from build123d import *

# Parameters (mm, degrees)
SKETCH_2_W               = 14
SKETCH_2_H               = 8
EXTRUDE_2_DEPTH          = 9
CUT_EXTRUDE_1_DEPTH      = 13.083045974
CUT_EXTRUDE_1_DEPTH_BACK = 13.083045974
SKETCH_3_R               = 1.35
SKETCH_3_2_R             = 1.35
EXTRUDE_3_DEPTH          = 3
SKETCH_6_R               = 1.5
CUT_EXTRUDE_3_DEPTH      = 10
SKETCH_7_R               = 4.5
CUT_EXTRUDE_4_DEPTH      = 4


with BuildPart() as part:
    # Sketch 2 → Extrude 2 (new, symmetric)
    with BuildSketch(Plane.XY):
        Rectangle(SKETCH_2_W, SKETCH_2_H)
    extrude(amount=EXTRUDE_2_DEPTH, both=True)

    # Sketch 3 → Cut-Extrude 1 (cut, two sides: drawn at the far end of the back side and taken through both)
    with BuildSketch(Plane(origin=(0, 0, 0), x_dir=(0, 0, -1), z_dir=(1, 0, 0)).offset(-CUT_EXTRUDE_1_DEPTH_BACK)):
        with Locations((6, 0)):
            Circle(SKETCH_3_R)
        with Locations((-6, 0)):
            Circle(SKETCH_3_R)
    extrude(amount=CUT_EXTRUDE_1_DEPTH + CUT_EXTRUDE_1_DEPTH_BACK, mode=Mode.SUBTRACT)

    # Sketch 3_2 → Extrude 3 (add, symmetric)
    with BuildSketch(Plane(origin=(0, 0, 0), x_dir=(0, 0, -1), z_dir=(1, 0, 0))):
        with Locations((6, 0)):
            Circle(SKETCH_3_2_R)
        with Locations((-6, 0)):
            Circle(SKETCH_3_2_R)
    extrude(amount=EXTRUDE_3_DEPTH, both=True)

    # Sketch 6 → Cut-Extrude 3 (cut)
    with BuildSketch(Plane.XZ.offset(4)):
        with Locations(Location((0, 0, 0), (0, 0, 270))):
            Circle(SKETCH_6_R)
    extrude(amount=-CUT_EXTRUDE_3_DEPTH, mode=Mode.SUBTRACT)

    # Sketch 7 → Cut-Extrude 4 (cut)
    with BuildSketch(Plane.XZ.offset(-4)):
        with Locations(Location((0, 0, 0), (0, 0, 270))):
            Circle(SKETCH_7_R)
    extrude(amount=CUT_EXTRUDE_4_DEPTH, mode=Mode.SUBTRACT)


solid = part.part
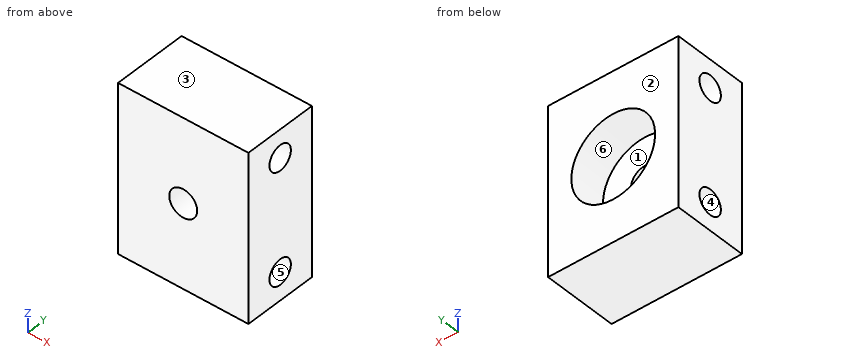
Read the model definition and answer for the solid it produces. Units are mm, in the model's axes. Face numbers are marked on the shaded views. A direction names the side the tool comes from. Give positions to 0.01 mm unless a question says otherwise; leave off trailing zeros. Write each loop counter-clockwise with the first axis right and the second up, starting at its lowest first coordinate (ties: lowest second). Pieces come first, ordered by that corner, then holes. Notation, with made-up numbers: (64.25, 7) - (85.25, 7) arc R13 cw to (85.25, 12) - close; hole circle Ø7 at (11, 50.5). An arc over 180 degrees is marked (long way). Use CSV: the item, a comma, the result in double quotes. Start each with the question number.
Item 1: For the marked faces 4, 5 and 6, determine the directions among +Z, -Z, +X, -X, +Y, -Y from which every point of the face is accessible in a straight line to the end or side of a thin tool.
Item 2: The part is cut by section C-C, the plane y = 2.5. Give the vertices of the cut face in (x, z).
Item 3: Flat-ended cylindrical pins translate along their axes: P1, Ø7, axis at x = 0, z = 0, coming from the -Y side; P2, Ø1.3, axis at y = 0, z = -6.5, coming from the +X side; P3, Ø2, axis at y = 0, z = -6, coming from the -X side. Find the tip coordinate at first contact, or state that the pin passes through.
Item 4: The part is cut by section B-B, the plane x = 0. Give the vertices of the cut face in (y, z), and give its area (3 significant figures).
Item 5: Consider line 1 (Z direction, x = 6.15, y = 0); line 2 (X direction, y = -0.5, z = 0); line 3 (Y direction, x = -5.3, z = 6). Determine where each line is inside the solid, lowest interval first.
Item 6: The part is cut by section D-D, the plane z = -6. Give the vertices of the cut face in (x, y).
Item 7: The part is cut by section A-A, the plane z = 0. Give the vertices of the cut face in (x, y).
Item 8: The mould has two halves that part along Z. Classify the marked faces 1, 2 and 3: pulls with the +Z half, pulls with the -Z half, needs draft (parallel to the pull), parting line crosses it, or undercut.
Taken from the geometry:
1,face 4,"-X"
1,face 5,"+X"
1,face 6,"+Y"
2,outline,"(-7, -9) - (7, -9) - (7, 9) - (-7, 9) - close; hole circle Ø9 at (0, 0)"
3,P1,"y = -4"
3,P2,"x = 3"
3,P3,"x = -3"
4,outline,"(-4, -9) - (4, -9) - (4, -4.5) - (0, -4.5) - (0, -1.5) - (-4, -1.5) - close; (-4, 1.5) - (0, 1.5) - (0, 4.5) - (4, 4.5) - (4, 9) - (-4, 9) - close"
4,area,"96.0 mm2"
5,line 1,"-9 to -7.35, -4.65 to 4.65, 7.35 to 9"
5,line 2,"-7 to -1.5, 1.5 to 7"
5,line 3,"-4 to -1.35, 1.35 to 4"
6,outline,"(-7, -4) - (7, -4) - (7, -1.35) - (3, -1.35) - (3, 1.35) - (7, 1.35) - (7, 4) - (-7, 4) - (-7, 1.35) - (-3, 1.35) - (-3, -1.35) - (-7, -1.35) - close"
7,outline,"(-7, -4) - (-1.5, -4) - (-1.5, 0) - (-4.5, 0) - (-4.5, 4) - (-7, 4) - close; (1.5, -4) - (7, -4) - (7, 4) - (4.5, 4) - (4.5, 0) - (1.5, 0) - close"
8,face 1,"undercut"
8,face 2,"needs draft"
8,face 3,"pulls with the +Z half"
